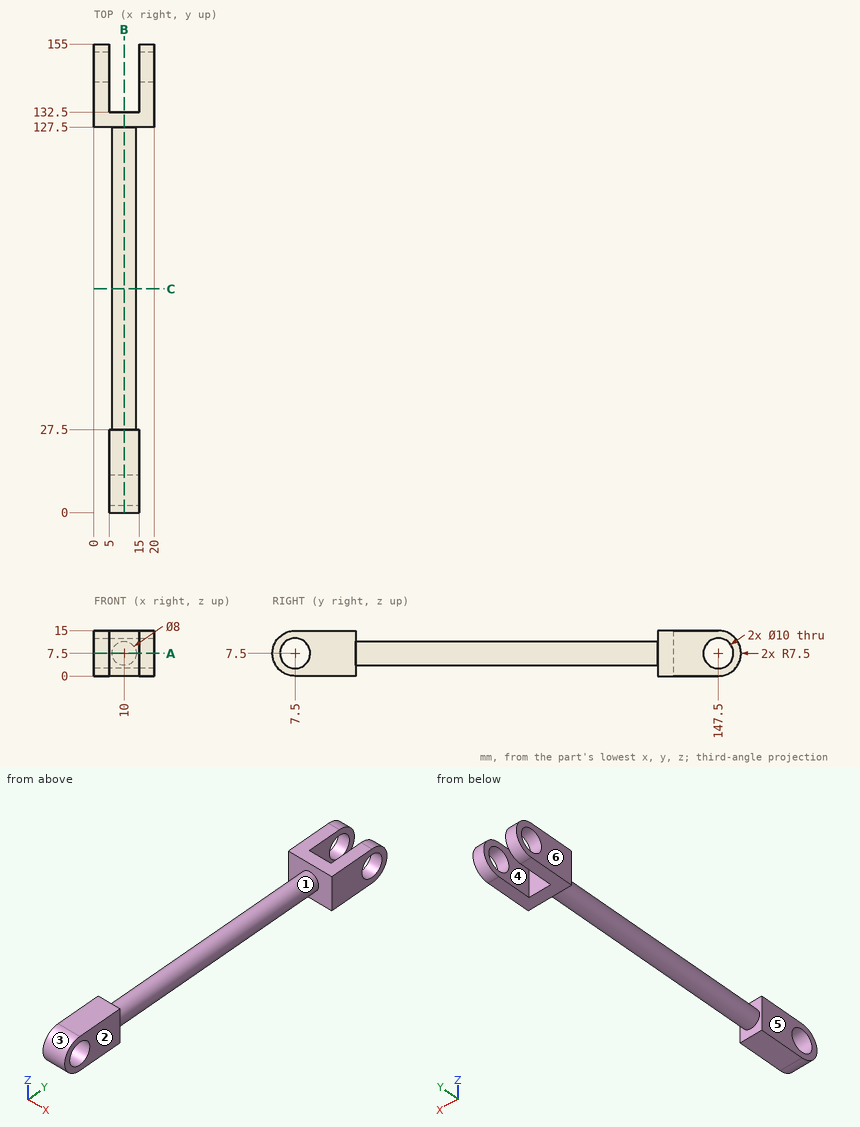
Study the drawing (mm; zero at the part's minimum x, y, z) and answer. A direction names the side the tool comes from. Give positions to 0.01 mm unless a question says otherwise; leave off trailing zeros. Order: outer loops, then holes, each group sorted by start corner. A loop starts at its lowest first (then second) coordinate and runs counter-clockwise, first axis right, second up. Notation, with made-up numbers: (1.5, -17) -> (33.5, -17) arc R17 ccw to (33.5, -4) -> close; hole circle Ø4 at (48.25, 73). An arc over 180 degrees is marked (long way). Put each result on its own line as item: value.
Item 1: For the marked faces 4, 5 and 6, determine the directions among +Z, -Z, +X, -X, +Y, -Y from which every point of the face is accessible in a straight line to the end or side of a thin tool.
Established:
face 4: +Z, -Z, +Y
face 5: +Z, -Z, -X, -Y
face 6: +Z, -Z, -X, +Y, -Y
Item 2: A cutting plane is placed at C-C on y = 74. Give the vertices of the cut face in (x, z), plus the area to 3 significant figures.
Established:
outline: circle Ø8 at (10, 7.5)
area: 50.3 mm^2
Item 3: For a pull along Y with two mould halves and no side action, classify the marked faces 1, 2 and 3 as released by +Y, released by -Y, zero draft, split by the parting line, or undercut.
Established:
face 1: undercut
face 2: zero draft
face 3: released by -Y
Item 4: A cutting plane is placed at B-B on x = 10. Give the vertices of the cut face in (y, z), plus the area to 3 significant figures.
Established:
outline: (7.5, 0) -> (27.5, 0) -> (27.5, 3.5) -> (127.5, 3.5) -> (127.5, 0) -> (132.5, 0) -> (132.5, 15) -> (127.5, 15) -> (127.5, 11.5) -> (27.5, 11.5) -> (27.5, 15) -> (7.5, 15) arc R7.5 ccw to start; hole circle Ø10 at (7.5, 7.5)
area: 1,180 mm^2
Item 5: Straight lines are drawn through the part: line 1 (Y direction, x = 6.75, z = 7); line 2 (Y direction, x = 1.45, z = 7.5); line 3 (Z direction, x = 18.3, y = 147.5). For each, find the intervals that lie inside material, in ascending order.
Established:
line 1: y = 0.02 to 2.53, 12.47 to 132.5
line 2: y = 127.5 to 142.5, 152.5 to 155
line 3: z = 0 to 2.5, 12.5 to 15
Item 6: Given P1, Ø5, axis at x = 8.5, z = 6.5, coming from the +Y side; P2, Ø2, axis at x = 11.5, z = 3.5, coming from the -Y side; P3, Ø3, axis at x = 7, y = 61, coming from the +Z side; P4, Ø7.5, axis at y = 140.5, z = 4, coming from the -X side, each flat-ended and moving along its own axis, determine where each tip first touches the part or whether it passes through.
Established:
P1: stops at y = 132.5
P2: stops at y = 0.63
P3: stops at z = 11.21
P4: stops at x = 0
Item 7: A cutting plane is placed at A-A on z = 7.5. Give the vertices of the cut face in (x, y), plus the area to 3 significant figures.
Established:
outline: (0, 127.5) -> (6, 127.5) -> (6, 27.5) -> (5, 27.5) -> (5, 12.5) -> (15, 12.5) -> (15, 27.5) -> (14, 27.5) -> (14, 127.5) -> (20, 127.5) -> (20, 142.5) -> (15, 142.5) -> (15, 132.5) -> (5, 132.5) -> (5, 142.5) -> (0, 142.5) -> close; (0, 152.5) -> (5, 152.5) -> (5, 155) -> (0, 155) -> close; (5, 0) -> (15, 0) -> (15, 2.5) -> (5, 2.5) -> close; (15, 152.5) -> (20, 152.5) -> (20, 155) -> (15, 155) -> close
area: 1,200 mm^2
